from build123d import *

# Parameters (mm, degrees)
F0_W     = 116.84
F0_H     = 17.78
F1_DEPTH = 15.24
F2_W     = 25.4
F2_H     = 17.78
F3_DEPTH = 10.16
F4_W     = 15.24
F4_H     = 25.4
F5_DEPTH = 25.4
F6_W     = 25.4
F6_H     = 25.4
F7_DEPTH = 25.4


with BuildPart() as f1:
    # F0 (on Right) → F1 (new body)
    with BuildSketch(Plane.YZ):
        with Locations((-0.526623, 44.730002)):
            Rectangle(F0_W, F0_H)
    extrude(amount=-F1_DEPTH)

    # F2 (on face) → F3 (join)
    with BuildSketch(Plane.YZ):
        with Locations((45.193377, 44.730002)):
            Rectangle(F2_W, F2_H)
    extrude(amount=F3_DEPTH)

    # F4 (on face) → F5 (join)
    with BuildSketch(Plane(origin=(0, 0, 35.840002), x_dir=(1, 0, 0), z_dir=(0, 0, -1))):
        with Locations((-7.62, 5.606623)):
            Rectangle(F4_W, F4_H)
    extrude(amount=F5_DEPTH)

    # F6 (on face) → F7 (join)
    with BuildSketch(Plane.YZ):
        with Locations((-5.606623, 23.140002)):
            Rectangle(F6_W, F6_H)
    extrude(amount=F7_DEPTH)


solid = f1.part
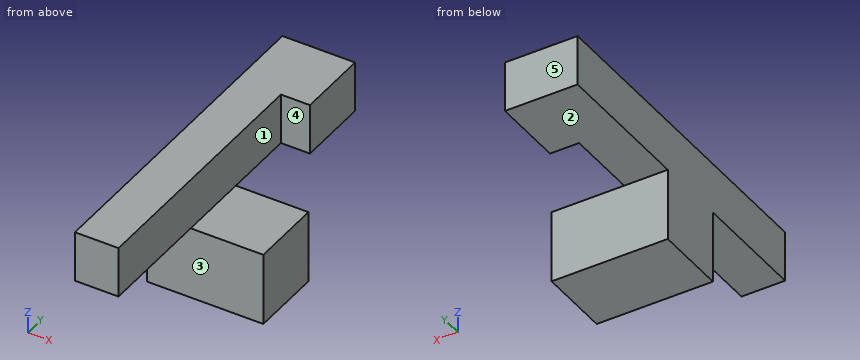
The listing builds one solid part. Answer for the finished solid, in the listing's coordinates (mm). Face numbers are marked on the shaded views. A direction names the side the tool comes from. Coordinates: 2 decimals unless noted, no trailing zeros. Loops run counter-clockwise (first coordinate to the right, second up) from the corner with the lowest first, then second, coordinate; pieces in that order, holes last.
1) Find section B-B on y = -8. Write down the section's boundary in (x, z).
2) Flat-ended cylindrical pins translate along their axes: pin 1 Ø7.5 at (x, y) = (18.5, -10.5) entering from +Z; pin 2 Ø12 at (x, z) = (-6.5, 25) entering from +Y; pin 3 Ø9 at (y, z) = (-22, 47) entering from +X; pin 4 Ø20.5 at (x, z) = (5.5, 28.5) entering from -Y. Find the tip coordinate at first contact, or state that the pin passes through.
3) Find section A-A on x = 8. Write down the section's boundary in (y, z).
4) A tool of negligible diameter and unlimited length cuts with its end or side. For the marked faces 1, 2, 3, 4 and 5, from which of +Z, -Z, +X, -X, +Y, -Y can it reach the whole face along a straight path? Write none if from no direction.
5) Find section C-C on x = -4. Write down the section's boundary in (y, z).
6) Find the intervals of material crossed by L1, parallel to Y at x = 9.5, z = 34.5; L2, parallel to Z at x = -12, y = 38; L3, parallel to X at y = -49.5, z = 40, in increasing order.
7) Find section D-D on z = 20. Write down the section's boundary in (x, y).
Values:
1. outline: (-15.24, 10.44) - (25.4, 10.44) - (25.4, 35.84) - (0, 35.84) - (0, 53.62) - (-15.24, 53.62) - close
2. pin 1: stops at z = 35.84
2. pin 2: stops at y = 7.09
2. pin 3: stops at x = 0
2. pin 4: stops at y = -58.95
3. outline: (-18.31, 10.44) - (7.09, 10.44) - (7.09, 35.84) - (-18.31, 35.84) - close; (32.49, 35.84) - (57.89, 35.84) - (57.89, 53.62) - (32.49, 53.62) - close
4. face 1: +Z, +X, -Y
4. face 2: -Z, +X, -X, +Y
4. face 3: -Z, +X, -X, -Y
4. face 4: +Z, -Z, +X, -Y
4. face 5: +Z, -Z, +X, -X, +Y
5. outline: (-58.95, 35.84) - (-18.31, 35.84) - (-18.31, 10.44) - (7.09, 10.44) - (7.09, 35.84) - (57.89, 35.84) - (57.89, 53.62) - (-58.95, 53.62) - close
6. L1: y = -18.31 to 7.09
6. L2: z = 35.84 to 53.62
6. L3: x = -15.24 to 0
7. outline: (-15.24, -18.31) - (25.4, -18.31) - (25.4, 7.09) - (-15.24, 7.09) - close
